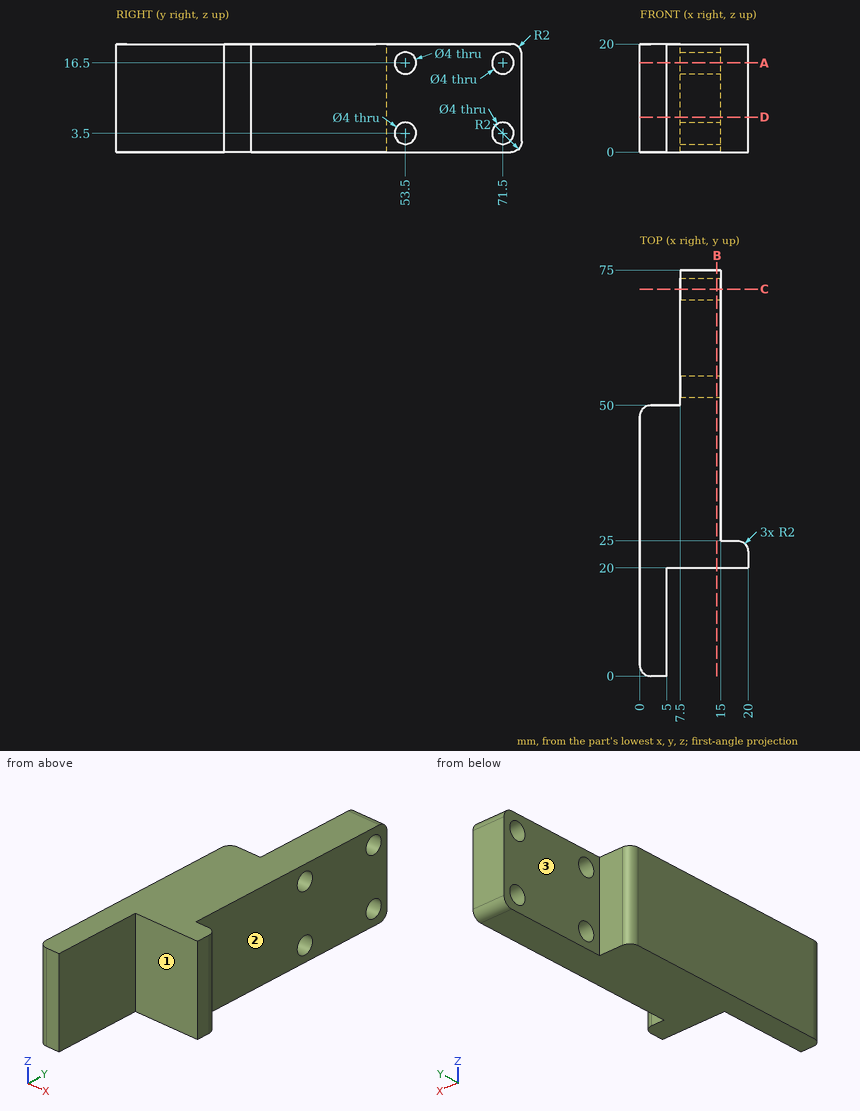
Part print with two shaded views. Sizes in mm from the minimum x, y, z corner. A direction names the side the tool comes from. Round coordinates to 2 decimals unless told otherwise and drop trailing zeros. Loops run counter-clockwise (first coordinate to the right, second up) from the corner with the lowest first, then second, coordinate; pieces in that order, holes last.
1. Slice it at C-C (y = 71.5). Give the cut face in (x, z), and give its area (3 significant figures).
Solutions:
outline: (7.5, 0) - (15, 0) - (15, 1.5) - (7.5, 1.5) - close; (7.5, 5.5) - (15, 5.5) - (15, 14.5) - (7.5, 14.5) - close; (7.5, 18.5) - (15, 18.5) - (15, 20) - (7.5, 20) - close
area: 90.0 mm2
2. Slice it at A-A (z = 16.5). Give the cut face in (x, y), and give its area (3 significant figures).
Solutions:
outline: (0, 2) arc R2 ccw to (2, 0) - (5, 0) - (5, 20) - (20, 20) - (20, 23) arc R2 ccw to (18, 25) - (15, 25) - (15, 51.5) - (7.5, 51.5) - (7.5, 50) - (2, 50) arc R2 ccw to (0, 48) - close; (7.5, 55.5) - (15, 55.5) - (15, 69.5) - (7.5, 69.5) - close; (7.5, 73.5) - (15, 73.5) - (15, 75) - (7.5, 75) - close
area: 700 mm2
3. Slice it at D-D (z = 6.5). Give the cut face in (x, y).
Solutions:
outline: (0, 2) arc R2 ccw to (2, 0) - (5, 0) - (5, 20) - (20, 20) - (20, 23) arc R2 ccw to (18, 25) - (15, 25) - (15, 75) - (7.5, 75) - (7.5, 50) - (2, 50) arc R2 ccw to (0, 48) - close
4. Flat gauge pins, fed straight in: pin 1 (4 mm diameter, centred on y = 63, z = 12.5, fed in from +X); pin 2 (2 mm diameter, centred on x = 5.5, z = 2.5, fed in from +Y); pin 3 (2.5 mm diameter, centred on y = 53.5, z = 16.5, fed in from -X); pin 4 (10 mm diameter, centred on y = 8.5, z = 10, fed in from +X). Where does each tip first touch, or does it go through?
Solutions:
pin 1: stops at x = 15
pin 2: stops at y = 50
pin 3: passes through
pin 4: stops at x = 5
5. 3-axis set-ups, long thin cutter, end or side, ignore diameter. For the marked faces 1, 2 and 3: which of +Z, -Z, +X, -X, +Y, -Y reach the whole face in a straight line?
Solutions:
face 1: +Z, -Z, +X, -Y
face 2: +Z, -Z, +X, +Y
face 3: +Z, -Z, -X, +Y
6. Slice it at B-B (x = 14.25). Give the cut face in (y, z), and give its area (3 significant figures).
Solutions:
outline: (20, 0) - (73, 0) arc R2 ccw to (75, 2) - (75, 18) arc R2 ccw to (73, 20) - (20, 20) - close; hole circle Ø4 at (53.5, 3.5); hole circle Ø4 at (53.5, 16.5); hole circle Ø4 at (71.5, 3.5); hole circle Ø4 at (71.5, 16.5)
area: 1,050 mm2
7. Drill centre lines: line 1 along Z through (x, y) = (13.5, 53.5); line 2 along Y through (x, z) = (11.5, 3.5); line 3 along Y through (x, z) = (14.75, 3). Where is each one in solid material? Low to high.
Solutions:
line 1: z = 0 to 1.5, 5.5 to 14.5, 18.5 to 20
line 2: y = 20 to 51.5, 55.5 to 69.5, 73.5 to 75
line 3: y = 20 to 51.56, 55.44 to 69.56, 73.44 to 75
